from build123d import *

# Parameters (mm, degrees)
SKETCH1_W           = 110
SKETCH1_H           = 150
BOSS_EXTRUDE1_DEPTH = 16
SKETCH4_W           = 110
SKETCH4_H           = 110
BOSS_EXTRUDE2_DEPTH = 20
SKETCH6_R           = 50
CUT_EXTRUDE1_DEPTH  = 10
FILLET1_R           = 50
SKETCH7_R           = 8
CUT_EXTRUDE4_DEPTH  = 194.971647413
SKETCH5_R           = 10
CUT_EXTRUDE5_DEPTH  = 2
CHAMFER3_SIZE       = 1
CHAMFER4_SIZE       = 1
CUT_EXTRUDE7_DEPTH  = 194.971647413
CHAMFER6_SIZE       = 3
FILLET3_R           = 3


with BuildPart() as part:
    # Sketch1 → Boss-Extrude1 (new body)
    with BuildSketch(Plane.XY):
        with Locations((0, 75)):
            Rectangle(SKETCH1_W, SKETCH1_H)
        with BuildLine():
            Line((-35.5, 135), (-35.5, 125))
            ThreePointArc((-35.5, 125), (-37.75, 122.75), (-40, 125))
            Line((-40, 125), (-40, 135))
            ThreePointArc((-40, 135), (-37.75, 137.25), (-35.5, 135))
        make_face(mode=Mode.SUBTRACT)
        with BuildLine():
            Line((35.5, 135), (35.5, 125))
            ThreePointArc((35.5, 125), (37.75, 122.75), (40, 125))
            Line((40, 125), (40, 135))
            ThreePointArc((40, 135), (37.75, 137.25), (35.5, 135))
        make_face(mode=Mode.SUBTRACT)
    extrude(amount=BOSS_EXTRUDE1_DEPTH)

    # Sketch4 → Boss-Extrude2 (add)
    with BuildSketch(Plane(origin=(0, 0, 0), x_dir=(1, 0, 0), z_dir=(0, 1, 0))):
        with Locations((0, -71)):
            Rectangle(SKETCH4_W, SKETCH4_H)
    extrude(amount=BOSS_EXTRUDE2_DEPTH)

    # Sketch6 → Cut-Extrude1 (cut)
    with BuildSketch(Plane(origin=(0, 20, 0), x_dir=(1, 0, 0), z_dir=(0, 1, 0))):
        with Locations(Location((0, -71, 0), (0, 0, 270))):
            Circle(SKETCH6_R)
    extrude(amount=-CUT_EXTRUDE1_DEPTH, mode=Mode.SUBTRACT)

    # Fillet1
    fillet1_edges = [part.edges().sort_by_distance(p)[0] for p in [
        (-55, 10, 126),
        (55, 10, 126),
    ]]
    fillet(fillet1_edges, radius=FILLET1_R)

    # Sketch7 → Cut-Extrude4 (cut, through all)
    with BuildSketch(Plane.XY.offset(16)):
        with Locations((0, 50)):
            Circle(SKETCH7_R)
    extrude(amount=-CUT_EXTRUDE4_DEPTH, mode=Mode.SUBTRACT)

    # Sketch5 → Cut-Extrude5 (cut)
    with BuildSketch(Plane.XY.offset(16)):
        with Locations((0, 50)):
            Circle(SKETCH5_R)
    extrude(amount=-CUT_EXTRUDE5_DEPTH, mode=Mode.SUBTRACT)

    # Chamfer3
    chamfer3_edges = [part.edges().sort_by_distance(p)[0] for p in [
        (0, 20, 16),
    ]]
    chamfer(chamfer3_edges, length=CHAMFER3_SIZE)

    # Chamfer4
    chamfer4_edges = [part.edges().sort_by_distance(p)[0] for p in [
        (0, 10, 21),
        (0, 20, 21),
    ]]
    chamfer(chamfer4_edges, length=CHAMFER4_SIZE)

    # Sketch8 → Cut-Extrude7 (cut, through all)
    with BuildSketch(Plane.XY.offset(16)):
        Polygon((-38.790019507, 98.174483069), (-10.505748259, 69.890211821), (-38.790019507, 41.605940574), align=None)
        Polygon((10.505748259, 69.890211821), (38.790019507, 41.605940574), (38.790019507, 98.174483069), align=None)
        Polygon((28.284271247, 109.186355869), (0, 80.902084621), (-28.284271247, 109.186355869), align=None)
    extrude(amount=-CUT_EXTRUDE7_DEPTH, mode=Mode.SUBTRACT)

    # Chamfer6
    chamfer6_edges = [part.edges().sort_by_distance(p)[0] for p in [
        (24.647883883, 84.032347445, 16),
        (24.647883883, 55.748076198, 16),
        (38.790019507, 69.890211821, 16),
        (0, 109.186355869, 16),
        (-14.142135624, 95.044220245, 16),
        (14.142135624, 95.044220245, 16),
        (-38.790019507, 69.890211821, 16),
        (-24.647883883, 55.748076198, 16),
        (-24.647883883, 84.032347445, 16),
    ]]
    chamfer(chamfer6_edges, length=CHAMFER6_SIZE)

    # Fillet3
    fillet3_edges = [part.edges().sort_by_distance(p)[0] for p in [
        (24.647883883, 55.748076198, 13),
        (38.790019507, 69.890211821, 13),
        (24.647883883, 84.032347445, 13),
        (-24.647883883, 55.748076198, 13),
        (-24.647883883, 84.032347445, 13),
        (-38.790019507, 69.890211821, 13),
        (-14.142135624, 95.044220245, 13),
        (14.142135624, 95.044220245, 13),
        (0, 109.186355869, 13),
    ]]
    fillet(fillet3_edges, radius=FILLET3_R)


solid = part.part
Here's how the part is built. I have some questions about the finished solid (model axes, mm). A direction names the side the tool comes from. Round coordinates to 2 decimals unless told otherwise and drop trailing zeros.
1. If we section it at A-A on x = -20: Count the separate pieces of the cut face and the enclosed holes in it, plus the area to 3 significant figures.
Answer list:
separate pieces: 3
enclosed holes: 0
area: 3,180 mm2
2. For P1, Ø4, axis at x = 34.5, z = 66, coming from the +Y side; P2, Ø12, axis at x = 36, z = 46.5, coming from the +Y side; P3, Ø12, axis at x = 13, y = 132, coming from the +Z side, each with a flat end and sliding along its axis, tell me the tip position at first contact or that it passes through.
Answer list:
P1: stops at y = 10
P2: stops at y = 10.55
P3: stops at z = 16
3. If I drill on line 1 along Y through (x, z) = (0, 3); line 2 along X through (y, z) = (13, 71); line 3 along Y through (x, z) = (5, 34), over which ranges is the centre line in solid material (lowest first)?
Answer list:
line 1: y = 0 to 42, 58 to 80.9, 109.19 to 150
line 2: x = -55 to -50, 50 to 55
line 3: y = 0 to 10
4. We'd pull the mould along Z, two halves only. Please class faces 5 (the face through (1, 10, 70)), 6 (the face through (24.54, 53.14, 14.92)), 7 (the face through (-24.846, 84.23, 5.961)): +Z half, -Z half, draft (parallel to the pull), parting line (faces both ways), or undercut.
Answer list:
face 5: undercut
face 6: +Z half
face 7: draft
5. Which directions (+Z, -Z, +X, -X, +Y, -Y) give clear straight access to the entire face, cutting with the end or side of a thin tool? Please do faces 1 (the face through (11, 86, 16)), 2 (the face through (35.5, 130, 8)), 3 (the face through (0, 58.2, 14)), 4 (the face through (-1, 0, 62)).
Answer list:
face 1: +Z, +X, -X, +Y
face 2: +Z, -Z
face 3: +Z
face 4: +Z, -Z, +X, -X, -Y
